Design review of the part built by this model. Coordinates are the model's own, in mm. A direction names the side the tool comes from. Coordinates: 2 decimals unless noted, no trailing zeros. Write each loop counter-clockwise with the first axis right and the second up, starting at its lowest first coordinate (ties: lowest second). Pieces come first, ordered by that corner, then holes. Notation, with made-up numbers: (31.25, 19) - (60.25, 19) arc R29 cw to (60.25, 42) - close; hole circle Ø1 at (61.25, -5). An arc over 180 degrees is marked (long way). Answer as a JSON object with one key per item and string values.
```python
from build123d import *

# Parameters (mm, degrees)
F1_DEPTH  = 3.175
F3_DEPTH  = 3.175
F6_W      = 50.8
F6_H      = 3.175
F9_W      = 25.4
F9_H      = 3.175
F12_R     = 3.96875
F13_DEPTH = 69.851


# Not quite as in the source:
# - a feature of the source that left no trace in its solid (it failed there, or was rolled back) is left out
# - a pattern or mirror of a feature is missing from the dataset's text; its kind, count and spacing are read off the source's solid


with BuildPart() as f1:
    # F0 (on Front) → F1 (new body)
    with BuildSketch(Plane.XZ):
        Polygon((0, 99.695), (0, 0), (63.5, 0), (63.5, 99.695), (50.8, 99.695), (50.8, 93.345), (12.7, 93.345), (12.7, 99.695), align=None)
    extrude(amount=F1_DEPTH)

    # F2 (on Right) → F3 (join)
    with BuildSketch(Plane.YZ):
        Polygon((-12.7, 0), (0, 0), (0, 99.695), (-12.7, 99.695), (-19.05, 93.345), (-19.05, 6.35), align=None)
    f3 = extrude(amount=-F3_DEPTH)

    # F3_copies: F3 across plane
    add(f3.mirror(Plane(origin=(31.75, 0, 0), x_dir=(0, 0, 1), z_dir=(1, 0, 0))))

    # F8: sweep along a path in F7
    with BuildLine(Plane.YZ) as f8_path:
        ThreePointArc((0, 0), (-2.7925061525, -3.6716217493), (-7.0765387245, -1.9610774491))
        Line((-7.0765387245, -1.9610774491), (-10.16, 3.175))
    # F6 (on face) → F8 (sweep)
    with BuildSketch(Plane(origin=(0, 0, 0), x_dir=(1, 0, 0), z_dir=(0, 0, -1))):
        with Locations((31.75, 1.5875)):
            Rectangle(F6_W, F6_H)
    sweep(path=f8_path.line)

    # F11: sweep along a path in F10
    with BuildLine(Plane.YZ) as f11_path:
        Line((-3.175, 93.345), (-12.7, 109.22))
    # F9 (on face) → F11 (sweep)
    with BuildSketch(Plane.XY.offset(93.345)):
        with Locations((31.75, -1.5875)):
            Rectangle(F9_W, F9_H)
    sweep(path=f11_path.line)

    # F12 (on face) → F13 (cut, through all)
    with BuildSketch(Plane(origin=(-3.175, 0, 0), x_dir=(0, -1, 0), z_dir=(-1, 0, 0))):
        with Locations((12.7, 86.995)):
            Circle(F12_R)
    extrude(amount=-F13_DEPTH, mode=Mode.SUBTRACT)


solid = f1.part
```
(1) Tool access review of faces 1 (the face through (31.57, -8, 101.39)), 2 (the face through (31.928, -4.829, 101.394)), 3 (the face through (1, -2, 99.695)): name each direction out of +Z, -Z, +X, -X, +Y, -Y from which nothing blocks a thin tool from reaching the whole face with its end or side.
Solved:
{"face 1": "-Y", "face 2": "+Z, +Y", "face 3": "+Z, -X, +Y, -Y"}
(2) For pin 1 (10 mm diameter, centred on x = 38.5, z = 47, fed in from -Y) (3 decimals); pin 2 (6 mm diameter, centred on x = 33, y = -3.5, fed in from +Z); pin 3 (3.5 mm diameter, centred on x = 46.5, y = -1.5, fed in from +Z) (3 decimals), all flat-tipped, find the tip position at first contact; note any pin that passes through.
Solved:
{"pin 1": "stops at y = -3.175", "pin 2": "stops at z = 104.18", "pin 3": "stops at z = 93.345"}
(3) Take a section at A-A, the plane x = 54.5. Write out the cut boundary in (y, z) (3 decimals), and give its area (3 significant figures).
Solved:
{"outline": "(-10.16, 3.175) - (-7.077, -1.961) arc R3.81 ccw to (0, 0) - (0, 99.695) - (-3.175, 99.695) - (-3.175, 0) arc R0.635 cw to (-4.354, -0.327) - (-7.438, 4.809) - close", "area": "354 mm^2"}
(4) The part is to be moulded in two halves that separate along X. For faces 4 (the face through (32.11, -5.92, 2.28)), 5 (the face through (31, 0, 49)), 6 (the face through (-3.175, -10, 51)), 7 (the face through (31.39, -8.82, 3.98)), say which applies: pulls with the +X half, pulls with the -X half, needs draft (parallel to the pull), parting line crosses it, or undercut.
Solved:
{"face 4": "undercut", "face 5": "needs draft", "face 6": "pulls with the -X half", "face 7": "undercut"}
(5) Take a section at B-B, the plane y = -6. Write out the cut boundary in (x, z) (3 decimals), and give its area (3 significant figures).
Solved:
{"outline": "(-3.175, 0) - (0, 0) - (0, 99.695) - (-3.175, 99.695) - close; (6.35, -3.118) - (57.15, -3.118) - (57.15, 2.414) - (6.35, 2.414) - close; (19.05, 98.053) - (44.45, 98.053) - (44.45, 103.345) - (19.05, 103.345) - close; (63.5, 0) - (66.675, 0) - (66.675, 99.695) - (63.5, 99.695) - close", "area": "1,050 mm^2"}
(6) To check wall thickness, follow line 1 (X direction, y = -8.5, z = 3) (3 decimals); line 2 (X direction, y = -14, z = 50.5) (3 decimals); line 3 (Z direction, x = 65, y = -12.7) (3 decimals). State the ranges of each line that lie inside material, in increasing order. Write a range as from..to.
Solved:
{"line 1": "x = -3.175..0, 6.35..57.15, 63.5..66.675", "line 2": "x = -3.175..0, 63.5..66.675", "line 3": "z = 0..83.026, 90.964..99.695"}
(7) Take a section at C-C, the plane z = 50. Write out the cut boundary in (x, y) (3 decimals), and give its area (3 significant figures).
Solved:
{"outline": "(-3.175, -19.05) - (0, -19.05) - (0, -3.175) - (63.5, -3.175) - (63.5, -19.05) - (66.675, -19.05) - (66.675, 0) - (-3.175, 0) - close", "area": "323 mm^2"}
(8) Take a section at D-D, the plane x = 41. Write out the cut boundary in (y, z) (3 decimals).
Solved:
{"outline": "(-12.7, 109.22) - (-3.175, 93.345) - (-3.175, 0) arc R0.635 cw to (-4.354, -0.327) - (-7.438, 4.809) - (-10.16, 3.175) - (-7.077, -1.961) arc R3.81 ccw to (0, 0) - (0, 93.345) - (-9.525, 109.22) - close"}
